Source: three-view drawing plus pictorial views. Frame: mm from the lowest corner of the part. A direction names the side the tool comes from. Give positions to 0.01 mm unless a question says otherwise; leave off trailing zeros. Loops run counter-clockwise (first coordinate to the right, second up) from the corner with the lowest first, then second, coordinate; pieces in that order, holes last. Notation, with made-up numbers: (73.25, 50.5) - (107.25, 50.5) arc R11 cw to (107.25, 71.5) - close; hole circle Ø7 at (-33, 63). An arc over 180 degrees is marked (long way). Answer as a JSON object with one key per item and string values.
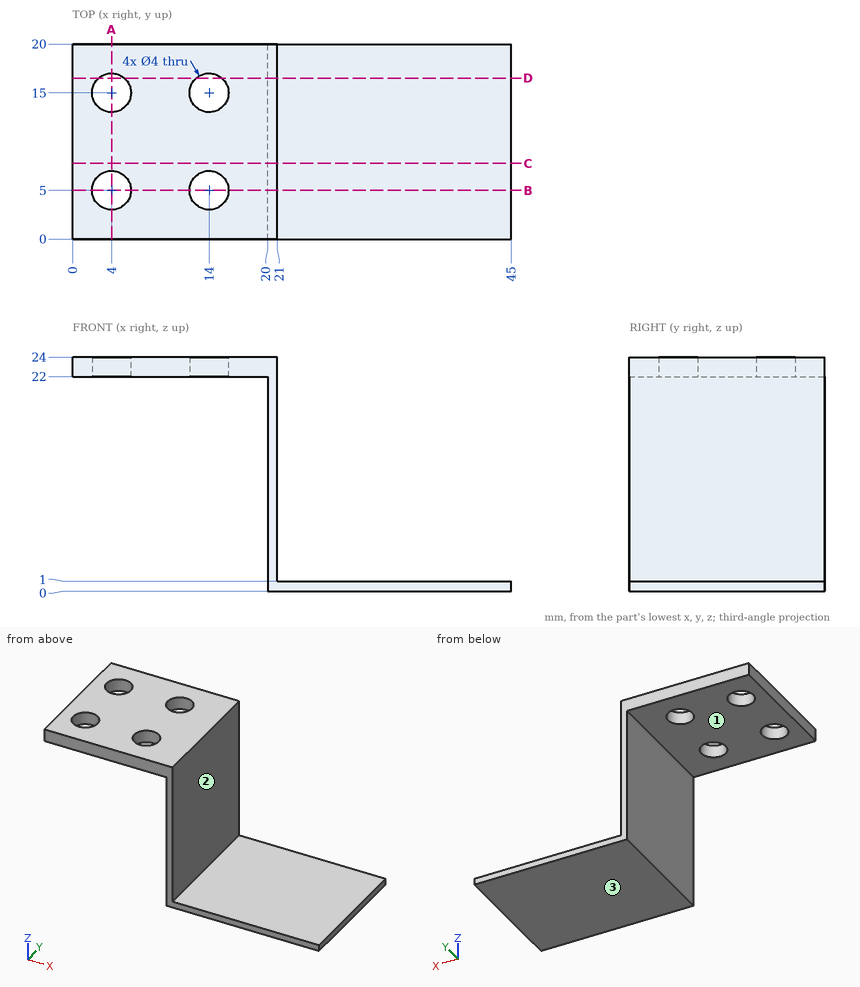
Item 1: Contact query for flat-ended pins moving along their axis: P1, Ø1, axis at y = 7, z = 15, coming from the -X side; P2, Ø10, axis at x = 37, y = 8, coming from the -Z side; P3, Ø4.5, axis at x = 4, y = 15, coming from the -Z side; P4, Ø1, axis at y = 3.5, z = 16, coming from the +X side. Output: stop coordinate, or through.
Geometry check:
{"P1": "stops at x = 20", "P2": "stops at z = 0", "P3": "stops at z = 22", "P4": "stops at x = 21"}
Item 2: Cut plane A-A (x = 4). Return loops of the section in (y, z).
Geometry check:
{"outline": "(0, 22) - (3, 22) - (3, 24) - (0, 24) - close; (7, 22) - (13, 22) - (13, 24) - (7, 24) - close; (17, 22) - (20, 22) - (20, 24) - (17, 24) - close"}
Item 3: Material intervals for line 1 (X direction, y = 5, z = 22.55); line 2 (Y direction, x = 4, z = 22.85); line 3 (Z direction, x = 30, y = 14.5), sorted ascending. Write a range as [from, to].
Geometry check:
{"line 1": "x = [0, 2], [6, 12], [16, 21]", "line 2": "y = [0, 3], [7, 13], [17, 20]", "line 3": "z = [0, 1]"}
Item 4: Cut plane D-D (y = 16.5). Return loops of the section in (x, z), then the cut area to 3 significant figures.
Geometry check:
{"outline": "(0, 22) - (2.68, 22) - (2.68, 24) - (0, 24) - close; (5.32, 22) - (12.68, 22) - (12.68, 24) - (5.32, 24) - close; (15.32, 22) - (20, 22) - (20, 0) - (45, 0) - (45, 1) - (21, 1) - (21, 24) - (15.32, 24) - close", "area": "77.4 mm2"}
Item 5: Cut plane C-C (y = 7.75). Return loops of the section in (x, z), then the cut area to 3 significant figures.
Geometry check:
{"outline": "(0, 22) - (20, 22) - (20, 0) - (45, 0) - (45, 1) - (21, 1) - (21, 24) - (0, 24) - close", "area": "88.0 mm2"}
Item 6: Cut plane B-B (y = 5). Return loops of the section in (x, z).
Geometry check:
{"outline": "(0, 22) - (2, 22) - (2, 24) - (0, 24) - close; (6, 22) - (12, 22) - (12, 24) - (6, 24) - close; (16, 22) - (20, 22) - (20, 0) - (45, 0) - (45, 1) - (21, 1) - (21, 24) - (16, 24) - close"}
Item 7: Access query for the marked faces 1, 2 and 3. Directions: +Z, -Z, +X, -X, +Y, -Y. A direction counts if a zero-diameter tool reaches every point of the face in a straight line with its end or side. Return the directions, or none.
Geometry check:
{"face 1": "-Z, -X, +Y, -Y", "face 2": "+Z, +X, +Y, -Y", "face 3": "-Z, +X, -X, +Y, -Y"}
